Source: CAD feature listing. Evaluate the final solid. Frame: model axes, mm. A direction names the side the tool comes from. Give positions to 0.01 mm unless a question says otherwise; leave off trailing zeros. Loops run counter-clockwise (first coordinate to the right, second up) from the corner with the lowest first, then second, coordinate; pieces in that order, holes last. Notation, with made-up numbers: M 33.25,45 L 63.25,45 A22 ccw 63.25,78 Z; hole C 33,-25 d3. An arc over 180 degrees is marked long. Put each result on its own line as item: value.
from build123d import *

# Parameters (mm, degrees)
SKETCH170_W     = 180
SKETCH170_H     = 144
PAD047_DEPTH    = 10
FILLET026_R     = 10
CHAMFER012_SIZE = 6
SKETCH171_R     = 2
POCKET058_DEPTH = 5


with BuildPart() as part:
    # Sketch170 → Pad047 (new body)
    with BuildSketch(Plane.XZ):
        Rectangle(SKETCH170_W, SKETCH170_H)
    extrude(amount=PAD047_DEPTH)

    # Fillet026
    fillet026_edges = [part.edges().sort_by_distance(p)[0] for p in [
        (-90, -5, 72),
        (90, -5, 72),
        (90, -5, -72),
        (-90, -5, -72),
    ]]
    fillet(fillet026_edges, radius=FILLET026_R)

    # Chamfer012
    chamfer012_edges = [part.edges().sort_by_distance(p)[0] for p in [
        (0, -10, 72),
        (90, -10, 0),
        (0, -10, -72),
        (-90, -10, 0),
    ]]
    chamfer(chamfer012_edges, length=CHAMFER012_SIZE)

    # Sketch171 (on Face4 of Chamfer012) → Pocket058 (cut)
    with BuildSketch(Plane(origin=(0, 0, 0), x_dir=(1, 0, 0), z_dir=(0, 1, 0))):
        with Locations((-80, -66)):
            Circle(SKETCH171_R)
        with Locations((-80, 45)):
            Circle(SKETCH171_R)
        with Locations((82.5, 43)):
            Circle(SKETCH171_R)
        with Locations((82.5, -47)):
            Circle(SKETCH171_R)
    extrude(amount=-POCKET058_DEPTH, mode=Mode.SUBTRACT)


with BuildPart() as part_1:
    # Body017 placement: moved
    add(part.part.moved(Location((-113, -183, 0))))


solid = part_1.part
1. Section query C-C (y = -191.25). Output: boundary loops of the cut face in (x, z), plus the area to 3 significant figures.
Found:
outline: M -198.75,-62 A5.75 ccw -193,-67.75 L -33,-67.75 A5.75 ccw -27.25,-62 L -27.25,62 A5.75 ccw -33,67.75 L -193,67.75 A5.75 ccw -198.75,62 Z
area: 23,200 mm^2
2. Contact query for flat-ended pins moving along their axis: P1, Ø1.2, axis at x = -192.5, z = -44.5, coming from the +Y side; P2, Ø6, axis at x = -144.5, y = -191, coming from the +Z side; P3, Ø1, axis at y = -188.5, z = -34.5, coming from the -X side. Output: stop coordinate, or through.
Found:
P1: y = -188
P2: z = 71
P3: x = -202
3. Draft query along X for faces 1 (the cylindrical face through (-194.474, -185.465, 64.648)), 2 (the flat face through (-114, -190, 69)), 3 (the flat face through (-23, -185, -1)). Return one class per face: pulls with the +X half, pulls with the -X half, needs draft (parallel to the pull), parting line crosses it, or undercut.
Found:
face 1: undercut
face 2: needs draft
face 3: pulls with the +X half
4. Access query for faces 4 (the conical face through (-28.44, -190.62, -66.46)), 5 (the cylindrical face through (-194.6, -185.5, -43.8)). Directions: +Z, -Z, +X, -X, +Y, -Y. A direction counts if a zero-diameter tool reaches every point of the face in a straight line with its end or side. Return the directions, or none.
Found:
face 4: -Z, +X, -Y
face 5: +Y
5. Material intervals for line 1 (Z direction, x = -193, y = -186.1); line 2 (Z direction, x = -30.5, y = -185.25); line 3 (X direction, y = -184.6, z = 47), sorted ascending. Write a range as from..to.
Found:
line 1: -72..-47, -43..64, 68..72
line 2: -71.68..-45, -41..45, 49..71.68
line 3: -203..-32.5, -28.5..-23
6. Section query B-B (x = -105). Output: boundary loops of the cut face in (y, z), plus the area to 3 significant figures.
Found:
outline: M -193,-66 L -187,-72 L -183,-72 L -183,72 L -187,72 L -193,66 Z
area: 1,400 mm^2
7. Section query A-A (z = -26). Output: boundary loops of the cut face in (x, y).
Found:
outline: M -203,-187 L -197,-193 L -29,-193 L -23,-187 L -23,-183 L -203,-183 Z
